Build history of the part. All positions in model axes, mm. Face numbers are marked on the shaded views. Round coordinates to 2 decimals unless told otherwise and drop trailing zeros. Write each loop counter-clockwise with the first axis right and the second up, starting at its lowest first coordinate (ties: lowest second). Pieces come first, ordered by that corner, then holes.
1) Saw through at A-A (y = 0). Write the cut outline in (x, z).
2) Wall check: probe 1 along Z at (x, y) = (21.25, -79.5); probe 2 along Z at (x, y) = (20.5, -69); probe 3 along Z at (x, y) = (5, -35). Give the ranges that are in metal, low to high.
3) Pull direction Z, two halves, no side cores. Call the marked faces 1, 2 and 3: +Z half, -Z half, draft (parallel to the pull), parting line (faces both ways), or undercut.
4) Flat gauge pins, fed straight in: pin 1 (16 mm diameter, centred on y = -30.61, z = -73.91, fed in from +X); pin 2 (8 mm diameter, centred on x = 4, z = -8, fed in from +Y); pin 3 (5 mm diameter, centred on x = 17.5, y = 50.5, fed in from -Z); pin 4 (1 mm diameter, centred on x = 17.5, z = 13.5, fed in from -Y). Where does each tip first touch, or does it go through?
5) Saw through at D-D (z = 77.5). Write the cut outline in (x, y).
6) Saw through at C-C (y = -36.5). Write the cut outline in (x, z).
Autodesk Inventor part; units mm, degrees
ref_plane "YZ Plane" through (0, 0, 0) normal (1, 0, 0) x (0, 1, 0)
ref_plane "XZ Plane" through (0, 0, 0) normal (0, 1, 0) x (-1, 0, 0)
ref_plane "XY Plane" through (0, 0, 0) normal (0, 0, 1) x (1, 0, 0)
sketch "Sketch1" plane through (0, 0, 0) normal (0, 0, 1) x (1, 0, 0)
  line L0 (24, 100) -> (0, 100)
  line L1 (0, 100) -> (0, 45.25)
  line L2 (0, 45.25) -> (0, 0) construction
  line L3 (0, 0) -> (24, 0) construction
  line L4 (24, 100) -> (24, 45.25)
  line L5 (24, 45.25) -> (0, 45.25)
  line L6 (24, 45.25) -> (24, 0) construction
  dimension "d0" = 200
  dimension "d1" = 24
  dimension "d5" = 90.5
revolve "Revolution1" add sketch "Sketch1" angle 360 about axis through (0, 0, 0) along (1, 0, 0)
sketch "Sketch2" plane through (0, 0, 0) normal (-1, 0, 0) x (0, 0, 1)
  circle A0 centre (0, 0) radius 45.25
  line L0 (0, 80) -> (0, 0) construction
  circle A1 centre (0, 0) radius 100
  circle A2 centre (0, 0) radius 80 construction
  line L1 (0, 0) -> (30.6147, 73.9104) construction
  circle A3 centre (30.6147, 73.9104) radius 9
  dimension "d6" = 18
  dimension "d7" = 80
  dimension "d8" = 22.5
extrude "Extrusion1" cut sketch "Sketch2" against normal through all contours A3
pattern_circular "Circular Pattern1" count 8 over 360 about axis through (12, 0, 0) along (1, 0, 0) of "Extrusion1"
equation "\"d6\" = dd2"
equation "\"d7\" = 0.5 * k"
equation "\"d0\" = D"
equation "\"d1\" = b"
equation "\"d5\" = dd5"
equation "\"b\" = 24"
equation "\"D\" = 200"
equation "\"dd2\" = 18"
equation "\"dd5\" = 90.5"
equation "\"Size_Designation\" = 1.2345"
properties part number "DIN EN 1092-1 Plate Flange for Welding Type 01 - PN 25 80 x 88.9" material "Steel"
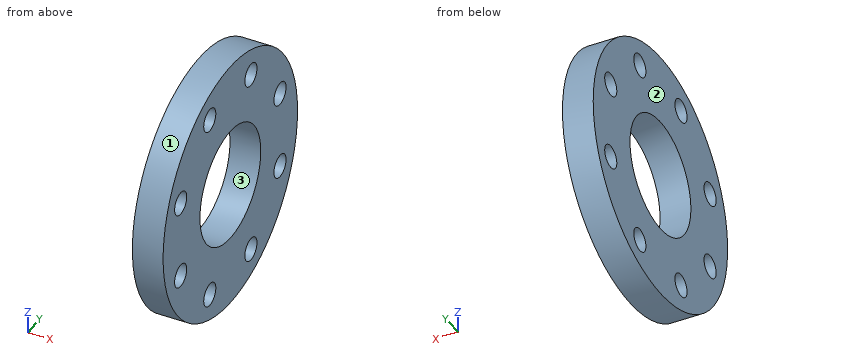
Evaluation:
1. outline: (0, -100) - (24, -100) - (24, -45.25) - (0, -45.25) - close; (0, 45.25) - (24, 45.25) - (24, 100) - (0, 100) - close
2. probe 1: z = -60.66 to -37.67, -23.56 to 23.56, 37.67 to 60.66
2. probe 2: z = -72.38 to -38.16, -23.07 to 23.07, 38.16 to 72.38
2. probe 3: z = -93.67 to -81.77, -66.05 to -28.68, 28.68 to 66.05, 81.77 to 93.67
3. face 1: parting line
3. face 2: draft
3. face 3: undercut
4. pin 1: passes through
4. pin 2: stops at y = 99.92
4. pin 3: stops at z = -87.73
4. pin 4: stops at y = -99.15
5. outline: (0, -63.2) - (24, -63.2) - (24, -38.87) - (0, -38.87) - close; (0, -22.36) - (24, -22.36) - (24, 22.36) - (0, 22.36) - close; (0, 38.87) - (24, 38.87) - (24, 63.2) - (0, 63.2) - close
6. outline: (0, -93.1) - (24, -93.1) - (24, -80.72) - (0, -80.72) - close; (0, -67.1) - (24, -67.1) - (24, -26.75) - (0, -26.75) - close; (0, 26.75) - (24, 26.75) - (24, 67.1) - (0, 67.1) - close; (0, 80.72) - (24, 80.72) - (24, 93.1) - (0, 93.1) - close
